Model file for the job. Use its own axes, mm. A direction names the side the tool comes from. Give positions to 0.01 mm unless a question says otherwise; leave off trailing zeros. Loops run counter-clockwise (first coordinate to the right, second up) from the corner with the lowest first, then second, coordinate; pieces in that order, holes last. Notation, with made-up numbers: M 51,66.25 L 107,66.25 A20 cw 107,94.25 Z; hole C 26,65.5 d2. An arc over 180 degrees is marked long. Use CSV: the item, a comma, the result in double quotes. Start each with the question number.
(1) Slice it at B-B on y = -4.25. List the corners of the cut face in (x, z), and give its area (3 significant figures).
(2) Slice it at A-A on z = 9.5. List the corners of the cut face in (x, y), and give its area (3 significant figures).
(3) Slice it at C-C on x = 10. List the corners of the cut face in (y, z).
(4) Two-plate mould, pull along Z, no slides. Class faces 1 (the face through (19.014, 4.965, 12.358)), 2 (the face through (0, 1, 8)), 3 (the face through (10, -5, 5)): pulls with the +Z half, pulls with the -Z half, needs draft (parallel to the pull), parting line crosses it, or undercut.
(5) Tool access for faces 4 (the face through (2, 2, 9)), 5 (the face through (20, 1, 8)), 6 (the face through (10, 12.823, 2)), 7 (the face through (12.65, -5, 10)), 8 (the face through (12.65, 3, 2)): list every direction of +Z, -Z, +X, -X, +Y, -Y with a clear straight run to the whole face (end or side of a thin tool).
(6) Wall check: line 1 along X through (y, z) = (-2.25, 6.75); line 2 along X through (y, z) = (-5.75, 10.5); line 3 along Z through (x, y) = (3.25, 9.5). Give the ranges that are in metal, low to high. Write a range as from..to.
(7) Slice it at D-D on z = 3.75. List the corners of the cut face in (x, y), and give its area (3 significant figures).
(8) Flat gauge pins, fed straight in: P1, Ø4.5, axis at x = 11, z = 9, coming from the +Y side; P2, Ø3, axis at x = 9.5, y = 4.5, coming from the -Z side; P3, Ø6, axis at x = 6, y = 9, coming from the +Z side. Where does each tip first touch, or does it go through?
```python
from build123d import *

# Parameters (mm, degrees)
SKETCH1_W           = 20
SKETCH1_H           = 20
BOSS_EXTRUDE1_DEPTH = 4.5
SKETCH2_W           = 20
SKETCH2_H           = 4.5
BOSS_EXTRUDE2_DEPTH = 4.5
BOSS_EXTRUDE3_DEPTH = 2


with BuildPart() as part:
    # Sketch1 → Boss-Extrude1 (new body)
    with BuildSketch(Plane.XY):
        with Locations((10, 2.82300885)):
            Rectangle(SKETCH1_W, SKETCH1_H)
        with BuildLine():
            Line((7.35, 5.17300885), (7.35, 0.47300885))
            ThreePointArc((7.35, 0.47300885), (10, -2.17699115), (12.65, 0.47300885))
            Line((12.65, 0.47300885), (12.65, 5.17300885))
            ThreePointArc((12.65, 5.17300885), (10, 7.82300885), (7.35, 5.17300885))
        make_face(mode=Mode.SUBTRACT)
    extrude(amount=BOSS_EXTRUDE1_DEPTH)

    # Sketch2 → Boss-Extrude2 (add)
    with BuildSketch(Plane.XZ.offset(7.17699115)):
        with Locations((10, 2.25)):
            Rectangle(SKETCH2_W, SKETCH2_H)
        with BuildLine():
            Line((0, 10), (0, 4.5))
            Line((0, 4.5), (20, 4.5))
            Line((20, 4.5), (20, 10))
            Line((20, 10), (12.65, 10))
            Line((12.65, 10), (12.65, 7.65))
            ThreePointArc((12.65, 7.65), (10, 5), (7.35, 7.65))
            Line((7.35, 7.65), (7.35, 10))
            Line((7.35, 10), (0, 10))
        make_face()
        with BuildLine():
            Line((0, 20), (0, 10))
            Line((0, 10), (7.35, 10))
            Line((7.35, 10), (7.35, 12.35))
            ThreePointArc((7.35, 12.35), (10, 15), (12.65, 12.35))
            Line((12.65, 12.35), (12.65, 10))
            Line((12.65, 10), (20, 10))
            Line((20, 10), (20, 20))
            Line((20, 20), (0, 20))
        make_face()
    extrude(amount=-BOSS_EXTRUDE2_DEPTH)

    # Sketch4 → Boss-Extrude3 (add)
    with BuildSketch(Plane(origin=(20, 0, 0), x_dir=(0, 0, -1), z_dir=(1, 0, 0))):
        Polygon((-20, -2.67699115), (-4.5, 12.82300885), (-4.5, -2.67699115), align=None)
    boss_extrude3 = extrude(amount=-BOSS_EXTRUDE3_DEPTH)

    # Mirror1: Boss-Extrude3 across plane
    add(boss_extrude3.mirror(Plane(origin=(10, 0, 0), x_dir=(0, 0, 1), z_dir=(1, 0, 0))))


solid = part.part
```
Reply:
1,outline,"M 0,0 L 20,0 L 20,20 L 0,20 Z; hole M 7.35,7.65 A2.65 ccw 12.65,7.65 L 12.65,12.35 A2.65 ccw 7.35,12.35 Z"
1,area,"353 mm^2"
2,outline,"M 0,-7.18 L 7.35,-7.18 L 7.35,-2.68 L 2,-2.68 L 2,7.82 L 0,7.82 Z; M 12.65,-7.18 L 20,-7.18 L 20,7.82 L 18,7.82 L 18,-2.68 L 12.65,-2.68 Z"
2,area,"108 mm^2"
3,outline,"M -7.18,0 L -2.18,0 L -2.18,4.5 L -2.68,4.5 L -2.68,5 L -7.18,5 Z; M -7.18,15 L -2.68,15 L -2.68,20 L -7.18,20 Z; M 7.82,0 L 12.82,0 L 12.82,4.5 L 7.82,4.5 Z"
4,face 1,"pulls with the +Z half"
4,face 2,"needs draft"
4,face 3,"undercut"
5,face 4,"+Z, +Y"
5,face 5,"+Z, -Z, +X, +Y, -Y"
5,face 6,"+Z, -Z, +X, -X, +Y"
5,face 7,"+Y, -Y"
5,face 8,"+Z, -Z"
6,line 1,"x = 0..2, 18..20"
6,line 2,"x = 0..7.35, 12.65..20"
6,line 3,"z = 0..4.5"
7,outline,"M 0,-7.18 L 20,-7.18 L 20,12.82 L 0,12.82 Z; hole M 7.35,0.47 A2.65 ccw 12.65,0.47 L 12.65,5.17 A2.65 ccw 7.35,5.17 Z"
7,area,"353 mm^2"
8,P1,"stops at y = -2.68"
8,P2,"passes through"
8,P3,"stops at z = 4.5"
